Verification items for the finished model (mm, model axes). A direction names the side the tool comes from. Coordinates: 2 decimals unless noted, no trailing zeros. Order: outer loops, then holes, each group sorted by start corner. A loop starts at its lowest first (then second) coordinate and runs counter-clockwise, first axis right, second up. Notation, with made-up numbers: (74, 2) -> (97, 2) arc R18 ccw to (97, 12) -> close; hole circle Ø9 at (-28, 29). An arc over 180 degrees is marked (long way). Write each question's results on one line, items separated by ' | '. Start each with the question number.
(1) Go/stop test with flat-tipped pins: pin 1 (1.2 mm diameter, centred on y = -0.5, z = 0, fed in from +X); pin 2 (1 mm diameter, centred on x = 21.5, z = -3, fed in from -Y); pin 3 (2 mm diameter, centred on y = 0, z = 0, fed in from +X); pin 4 (1 mm diameter, centred on x = 33, z = 0, fed in from +Y). Record where each tip stops, or that it passes through.
(2) Cross-section at A-A on x = 4.5. Enter the section's corners in (y, z).
(3) Draft check along Y on faces 3 (the cylindrical face through (17.941, 3.695, -1.532)), 4 (the flat face through (34.5, 1, 1)), 5 (the cylindrical face through (32.237, -2.292, 0.24)). Enter one of: +Y half, -Y half, draft (parallel to the pull), parting line (faces both ways), or undercut.
(4) Thickness scan on probe 1 along Y at (x, z) = (34.75, 0); probe 2 along Z at (x, y) = (32.35, 0); probe 3 along Z at (x, y) = (33, 1.4). Record the ranges inside material, lowest first. Write a range as [from, to].
(5) Set-up check for faces 1 (the cylindrical face through (32.237, 2.292, -0.24)), 2 (the cylindrical face through (32.98, -0.15, -1.14)): record each of +Z, -Z, +X, -X, +Y, -Y from which the full face is reachable in a straight line by a thin tool's end or side.
Autodesk Inventor part; units mm, degrees
ref_plane "YZ Plane" through (0, 0, 0) normal (1, 0, 0) x (0, 1, 0)
ref_plane "XZ Plane" through (0, 0, 0) normal (0, 1, 0) x (-1, 0, 0)
ref_plane "XY Plane" through (0, 0, 0) normal (0, 0, 1) x (1, 0, 0)
sketch "Sketch1" plane through (0, 0, 0) normal (0, 0, 1) x (1, 0, 0)
  line L0 (0, 0) -> (0, 3)
  line L1 (0, 3) -> (15, 3)
  line L2 (15, 3) -> (15, 4)
  line L3 (15, 4) -> (35, 4)
  line L4 (35, 4) -> (35, 0)
  line L5 (35, 0) -> (0, 0)
  line L6 (34.5, 0) -> (34.5, 2)
  line L7 (34.5, 2) -> (35, 2)
  line L8 (34.5, 1.15) -> (31.5, 1.15)
  line L9 (31.5, 1.15) -> (30.7814, 0)
  line L10 (30.7814, 0) -> (34.5, 0)
  line L11 (15, 4) -> (0, 4)
  line L12 (0, 4) -> (0, 3)
  point P0 (0, 1.5)
  point P1 (35, 2)
  dimension "d0" = 3
  dimension "d1" = 4
  dimension "d2" = 15
  dimension "d3" = 35
  dimension "d4" = 2
  dimension "d5" = 0.5
  dimension "d27" = 1.15
  dimension "d28" = 58
  dimension "d29" = 3
revolve "Revolution1" add sketch "Sketch1" angle 360 about axis through (35, 0, 0) along (-1, 0, 0) contours L0 L1 L2 L3 L4 L7 L6 L8 L9 L5 | L12 L11 L2 L1
chamfer "Chamfer1" [suppressed]
chamfer "Chamfer2" distance 0.1 angle 45 1 edges at (35, -4, 0)
sketch "Sketch2" plane through (0, 0, 0) normal (0, 1, 0) x (-1, 0, 0)
  circle A0 centre (-33, 0) radius 0.8
  line L0 (-35, -2) -> (-35, 2)
  point P0 (0, 0)
  dimension "d13" = 1.6
  dimension "d14" = 2
extrude "Extrusion1" cut sketch "Sketch2" along normal mid plane 10
chamfer "Chamfer4" distance 0.2 angle 45 3 edges at (33, 3.9192, 0.8) (33.0001, 3.9192, -0.8) (33.8, -4, 0.001)
thread "Thread2"
thread "Thread3"
chamfer "Chamfer5" distance 0.5 angle 45 1 edges at (0, -4, 0)
properties part number "Sp mu SM holder"
Results are:
1) pin 1: stops at x = 31.47 | pin 2: stops at y = -3.12 | pin 3: stops at x = 31.41 | pin 4: passes through
2) outline: circle Ø8 at (0, 0)
3) face 3: parting line | face 4: undercut | face 5: draft
4) probe 1: y = [-4, -2], [2, 4] | probe 2: z = [-4, -1.15], [1.15, 4] | probe 3: z = [-3.75, -0.8], [0.8, 3.75]
5) face 1: +Y, -Y | face 2: +X
